from build123d import *

# Parameters (mm, degrees)
SKETCH1_W           = 51.6
SKETCH1_H           = 26.6
BOSS_EXTRUDE1_DEPTH = 23.05
SKETCH2_W           = 45.6
SKETCH2_H           = 20.6
SKETCH2_W_2         = 11
SKETCH2_H_2         = 26.6
CUT_EXTRUDE1_DEPTH  = 4
SKETCH3_W           = 45.6
SKETCH3_H           = 20.6
CUT_EXTRUDE2_DEPTH  = 16.05
CUT_EXTRUDE3_DEPTH  = 3.1
SKETCH6_W           = 51.6
SKETCH6_H           = 3.1
BOSS_EXTRUDE2_DEPTH = 11
SKETCH7_W           = 51.6
SKETCH7_H           = 3.1
BOSS_EXTRUDE3_DEPTH = 11
SKETCH8_W           = 11
SKETCH8_H           = 26.6
CUT_EXTRUDE4_DEPTH  = 5
SKETCH9_W           = 51.6
SKETCH9_H           = 26.6
CUT_EXTRUDE5_DEPTH  = 5
BOSS_EXTRUDE4_DEPTH = 2


with BuildPart() as part:
    # Sketch1 → Boss-Extrude1 (new body)
    with BuildSketch(Plane.XY):
        with Locations((25.8, 13.3)):
            Rectangle(SKETCH1_W, SKETCH1_H)
    extrude(amount=BOSS_EXTRUDE1_DEPTH)

    # Sketch2 → Cut-Extrude1 (cut)
    with BuildSketch(Plane.XY.offset(23.05)):
        with Locations((25.8, 13.3)):
            Rectangle(SKETCH2_W, SKETCH2_H)
        with Locations((25.8, 13.3)):
            Rectangle(SKETCH2_W_2, SKETCH2_H_2)
    extrude(amount=-CUT_EXTRUDE1_DEPTH, mode=Mode.SUBTRACT)

    # Sketch3 → Cut-Extrude2 (cut)
    with BuildSketch(Plane.XY.offset(19.05)):
        with Locations((25.8, 13.3)):
            Rectangle(SKETCH3_W, SKETCH3_H)
    extrude(amount=-CUT_EXTRUDE2_DEPTH, mode=Mode.SUBTRACT)

    # Sketch4 → Cut-Extrude3 (cut)
    with BuildSketch(Plane(origin=(0, 0, 0), x_dir=(-1, 0, 0), z_dir=(0, 0, -1))):
        with BuildLine():
            ThreePointArc((-30.9, 13.3), (-33.243145751, 18.956854249), (-38.9, 21.3))
            Line((-38.9, 21.3), (-38.9, 13.3))
            Line((-38.9, 13.3), (-46.9, 13.3))
            ThreePointArc((-46.9, 13.3), (-38.9, 5.3), (-30.9, 13.3))
        make_face()
        with BuildLine():
            Line((-38.9, 13.3), (-38.9, 21.3))
            ThreePointArc((-38.9, 21.3), (-44.556854249, 18.956854249), (-46.9, 13.3))
            Line((-46.9, 13.3), (-38.9, 13.3))
        make_face()
        with BuildLine():
            ThreePointArc((-30.9, 13.3), (-33.243145751, 18.956854249), (-38.9, 21.3))
            Line((-38.9, 21.3), (-38.9, 13.3))
            Line((-38.9, 13.3), (-46.9, 13.3))
            ThreePointArc((-46.9, 13.3), (-38.9, 5.3), (-30.9, 13.3))
        make_face()
        with BuildLine():
            Line((-38.9, 13.3), (-38.9, 21.3))
            ThreePointArc((-38.9, 21.3), (-44.556854249, 18.956854249), (-46.9, 13.3))
            Line((-46.9, 13.3), (-38.9, 13.3))
        make_face()
        with BuildLine():
            ThreePointArc((-12.7, 21.3), (-18.356854249, 7.643145751), (-4.7, 13.3))
            Line((-4.7, 13.3), (-12.7, 13.3))
            Line((-12.7, 13.3), (-12.7, 21.3))
        make_face()
        with BuildLine():
            Line((-12.7, 13.3), (-4.7, 13.3))
            ThreePointArc((-4.7, 13.3), (-7.043145751, 18.956854249), (-12.7, 21.3))
            Line((-12.7, 21.3), (-12.7, 13.3))
        make_face()
        with BuildLine():
            ThreePointArc((-12.7, 21.3), (-18.356854249, 7.643145751), (-4.7, 13.3))
            Line((-4.7, 13.3), (-12.7, 13.3))
            Line((-12.7, 13.3), (-12.7, 21.3))
        make_face()
        with BuildLine():
            Line((-12.7, 13.3), (-4.7, 13.3))
            ThreePointArc((-4.7, 13.3), (-7.043145751, 18.956854249), (-12.7, 21.3))
            Line((-12.7, 21.3), (-12.7, 13.3))
        make_face()
    extrude(amount=-CUT_EXTRUDE3_DEPTH, mode=Mode.SUBTRACT)

    # Sketch6 → Boss-Extrude2 (add)
    with BuildSketch(Plane(origin=(0, 26.6, 0), x_dir=(1, 0, 0), z_dir=(0, 1, 0))):
        with Locations((25.8, -1.55)):
            Rectangle(SKETCH6_W, SKETCH6_H)
    extrude(amount=BOSS_EXTRUDE2_DEPTH)

    # Sketch7 → Boss-Extrude3 (add)
    with BuildSketch(Plane.XY.offset(3.1)):
        with Locations((25.8, 36.05)):
            Rectangle(SKETCH7_W, SKETCH7_H)
    extrude(amount=BOSS_EXTRUDE3_DEPTH)

    # Sketch8 → Cut-Extrude4 (cut)
    with BuildSketch(Plane.XY.offset(19.05)):
        with Locations((25.8, 13.3)):
            Rectangle(SKETCH8_W, SKETCH8_H)
    extrude(amount=-CUT_EXTRUDE4_DEPTH, mode=Mode.SUBTRACT)

    # Sketch9 → Cut-Extrude5 (cut)
    with BuildSketch(Plane.XY.offset(23.05)):
        with Locations((25.8, 13.3)):
            Rectangle(SKETCH9_W, SKETCH9_H)
    extrude(amount=-CUT_EXTRUDE5_DEPTH, mode=Mode.SUBTRACT)

    # Sketch10 → Boss-Extrude4 (add)
    with BuildSketch(Plane.XY.offset(18.05)):
        Polygon((0, 0), (20.3, 0), (20.3, 3), (3, 3), (3, 23.6), (20.3, 23.6), (20.3, 26.6), (0, 26.6), align=None)
        Polygon((31.3, 0), (51.6, 0), (51.6, 26.6), (31.3, 26.6), (31.3, 23.6), (48.6, 23.6), (48.6, 3), (31.3, 3), align=None)
    extrude(amount=BOSS_EXTRUDE4_DEPTH)


solid = part.part
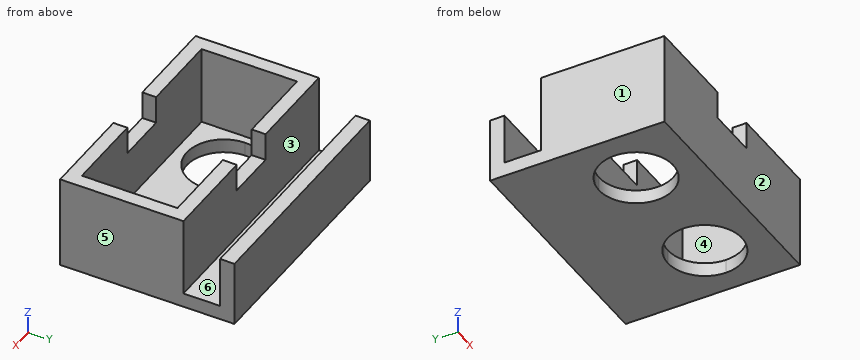
Geometry: final body of the model. Coordinates: model frame, mm. Face numbers are marked on the shaded views. A direction names the side the tool comes from. Coordinates: 2 decimals unless noted, no trailing zeros. Order: outer loops, then holes, each group sorted by start corner. A loop starts at its lowest first (then second) coordinate and runs counter-clockwise, first axis right, second up. Notation, with made-up numbers: M -13.5,11 L -3.5,11 A15 cw -3.5,30 Z; hole C 16.5,-29 d4. An arc over 180 degrees is marked long. One line per question, with ' | ' between items. Start each with the question number.
Item 1: Ray query, probe 1 along Y at (x, z) = (31, 12.25); probe 2 along X at (y, z) = (16, 17); probe 3 along Y at (x, z) = (36.5, 16.75). Return the intervals inside material, ascending. Write a range as [from, to].
Item 2: Cut plane C-C, the plane y = 10.5. Return the cut outline in (x, z).
Item 3: Draft query along Y for the marked faces 1, 2 and 3. Return one class per face: released by +Y, released by -Y, zero draft, split by the parting line, or undercut.
Item 4: Pin query (flat end, axial travel): pin 1 Ø16.5 at (x, y) = (23.5, 11.5) entering from +Z; pin 2 Ø3.5 at (x, y) = (24, 1) entering from +Z; pin 3 Ø4 at (x, y) = (26, 29.5) entering from +Z. Return the tip coordinate at first contact, or that it passes through.
Item 5: Cut plane A-A, the plane z = 11. Return the cut outline in (x, y), then the cut area to 3 significant figures.
Item 6: Set-up query: the marked faces 4, 5 and 6. Return all of +Z, -Z, +X, -X, +Y, -Y with unobstructed straight access to the full face (end or side cutting, diameter ignored); none if empty.
Item 7: Cut plane B-B, the plane x = 41. Return the cut outline in (y, z).
Item 8: Cut plane D-D, the plane x = 27.5. Return the cut outline in (y, z).
A:
1) probe 1: y = [0, 3], [23.6, 26.6], [34.5, 37.6] | probe 2: x = [0, 3], [48.6, 51.6] | probe 3: y = [0, 3], [23.6, 26.6]
2) outline: M 0,0 L 5.21,0 L 5.21,3 L 3,3 L 3,20.05 L 0,20.05 Z; M 20.19,0 L 31.41,0 L 31.41,3 L 20.19,3 Z; M 46.39,0 L 51.6,0 L 51.6,20.05 L 48.6,20.05 L 48.6,3 L 46.39,3 Z
3) face 1: zero draft | face 2: released by -Y | face 3: undercut
4) pin 1: stops at z = 3 | pin 2: stops at z = 14.05 | pin 3: stops at z = 3.1
5) outline: M 0,0 L 51.6,0 L 51.6,26.6 L 0,26.6 Z; M 0,34.5 L 51.6,34.5 L 51.6,37.6 L 0,37.6 Z; hole M 3,3 L 48.6,3 L 48.6,23.6 L 3,23.6 Z | area: 593 mm2
6) face 4: +Z | face 5: +Z, -Z, +X, +Y, -Y | face 6: +Z, +X, -X
7) outline: M 0,0 L 5.58,0 L 5.58,3 L 3,3 L 3,20.05 L 0,20.05 Z; M 21.02,0 L 37.6,0 L 37.6,14.1 L 34.5,14.1 L 34.5,3.1 L 26.6,3.1 L 26.6,20.05 L 23.6,20.05 L 23.6,3 L 21.02,3 Z
8) outline: M 0,0 L 37.6,0 L 37.6,14.1 L 34.5,14.1 L 34.5,3.1 L 26.6,3.1 L 26.6,14.05 L 23.6,14.05 L 23.6,3 L 3,3 L 3,14.05 L 0,14.05 Z
